Autodesk Inventor part; units mm, degrees
ref_plane "YZ Plane" through (0, 0, 0) normal (1, 0, 0) x (0, 1, 0)
ref_plane "XZ Plane" through (0, 0, 0) normal (0, 1, 0) x (-1, 0, 0)
ref_plane "XY Plane" through (0, 0, 0) normal (0, 0, 1) x (1, 0, 0)
sketch "Sketch1" plane through (0, 0, 0) normal (0, 0, 1) x (1, 0, 0)
  line L0 (20, 110) -> (0, 110)
  line L1 (0, 110) -> (0, 57.95)
  line L2 (0, 57.95) -> (0, 0) construction
  line L3 (0, 0) -> (20, 0) construction
  line L4 (20, 110) -> (20, 57.95)
  line L5 (20, 57.95) -> (0, 57.95)
  line L6 (20, 57.95) -> (20, 0) construction
  dimension "d0" = 220
  dimension "d1" = 20
  dimension "d5" = 115.9
revolve "Revolution1" add sketch "Sketch1" angle 360 about axis through (0, 0, 0) along (1, 0, 0)
sketch "Sketch2" plane through (0, 0, 0) normal (-1, 0, 0) x (0, 0, 1)
  circle A0 centre (0, 0) radius 57.95
  line L0 (0, 90) -> (0, 0) construction
  circle A1 centre (0, 0) radius 110
  circle A2 centre (0, 0) radius 90 construction
  line L1 (0, 0) -> (34.4415, 83.1492) construction
  circle A3 centre (34.4415, 83.1492) radius 9
  dimension "d6" = 18
  dimension "d7" = 90
  dimension "d8" = 22.5
extrude "Extrusion1" cut sketch "Sketch2" against normal through all contours A3
pattern_circular "Circular Pattern1" count 8 over 360 about axis through (10, 0, 0) along (1, 0, 0) of "Extrusion1"
equation "\"d6\" = dd2"
equation "\"d7\" = 0.5 * k"
equation "\"d0\" = D"
equation "\"d1\" = b"
equation "\"d5\" = dd5"
equation "\"b\" = 20"
equation "\"D\" = 220"
equation "\"dd2\" = 18"
equation "\"dd5\" = 115.9"
equation "\"Size_Designation\" = 1.2345"
properties part number "DIN 2576 Slip-On Flange for Welding Series 1 (ISO) - PN 10 100 x 114.3" material "Steel"
Here's how the part is built. I have some questions about the finished solid (model axes, mm). Coordinates: 2 decimals unless noted, no trailing zeros. Write each loop counter-clockwise with the first axis right and the second up, starting at its lowest first coordinate (ties: lowest second). Pieces come first, ordered by that corner, then holes.
1) Thinking about a two-plate mould opening in Y: for faces 1 (the face through (0, 47, -47)), 2 (the face through (9.86, 77.67, 27.3)), 3 (the face through (9.86, -30.28, -91.13)), 4 (the face through (9.86, -23.846, 107.384)), which applies, +Y half, -Y half, draft (parallel to the pull), parting line (faces both ways), or undercut?
Filled in:
face 1: draft
face 2: undercut
face 3: undercut
face 4: parting line
2) If we section it at A-A (y = 0): List the corners of the cut face in (x, z) for me, plus the area to 3 significant figures.
Filled in:
outline: (0, -110) - (20, -110) - (20, -57.95) - (0, -57.95) - close; (0, 57.95) - (20, 57.95) - (20, 110) - (0, 110) - close
area: 2,080 mm2
3) If we section it at C-C (x = 16.5): Count the separate pieces of the cut face and the enclosed holes in it, plus the area to 3 significant figures.
Filled in:
separate pieces: 1
enclosed holes: 9
area: 25,400 mm2
4) If I drill on line 1 (Y direction, x = 7.75, z = -34.5); line 2 (Z direction, x = 17.25, y = -34); line 3 (Z direction, x = 6, y = 86), over which ranges is the centre line in solid material (lowest first)?
Filled in:
line 1: y = -104.45 to -92.15, -74.15 to -46.56, 46.56 to 74.15, 92.15 to 104.45
line 2: z = -104.61 to -92.14, -74.16 to -46.93, 46.93 to 74.16, 92.14 to 104.61
line 3: z = -68.59 to -42.98, -25.9 to 25.9, 42.98 to 68.59
5) I'm going to push flat-ended pins straight in: pin 1 (8 mm diameter, centred on x = 8.5, y = 6, fed in from +Z); pin 2 (23.5 mm diameter, centred on y = 34.44, z = -83.15, fed in from +X); pin 3 (8 mm diameter, centred on x = 4, y = 64, fed in from +Z); pin 4 (11 mm diameter, centred on y = 34.44, z = 83.15, fed in from -X). Where does each tip first touch, or does it pass through?
Filled in:
pin 1: stops at z = 109.98
pin 2: stops at x = 20
pin 3: stops at z = 92.2
pin 4: passes through
